from build123d import *

# Parameters (mm, degrees)
SKETCH_4_W          = 160
SKETCH_4_H          = 115
EXTRUDE_1_DEPTH     = 20
CUT_EXTRUDE_1_DEPTH = 20
SKETCH_16_R         = 5.5
CUT_EXTRUDE_2_DEPTH = 15


with BuildPart() as part:
    # 草圖4 → 填料-伸長1 (new body)
    with BuildSketch(Plane.XY):
        with Locations((14.659712787, 72.59909222)):
            Rectangle(SKETCH_4_W, SKETCH_4_H)
    extrude(amount=EXTRUDE_1_DEPTH)

    # 草圖2 → 除料-伸長1 (cut)
    with BuildSketch(Plane.XY):
        with BuildLine():
            Line((9.582154386, 114.239387395), (32.639572719, 114.239387395))
            Line((32.639572719, 114.239387395), (35.911975242, 114.239387395))
            Line((35.911975242, 114.239387395), (35.911975242, 122.748829131))
            Line((35.911975242, 122.748829131), (43.825042281, 122.748829131))
            Line((43.825042281, 122.748829131), (43.825042281, 116.150572029))
            Line((43.825042281, 116.150572029), (45.365452665, 116.150572029))
            Line((45.365452665, 116.150572029), (45.365452665, 126.787374199))
            Line((45.365452665, 126.787374199), (50.650153823, 126.787374199))
            Line((50.650153823, 126.787374199), (50.650153823, 116.150572029))
            Line((50.650153823, 116.150572029), (51.63260176, 116.150572029))
            Line((51.63260176, 116.150572029), (51.63260176, 122.748829131))
            Line((51.63260176, 122.748829131), (58.302252446, 122.748829131))
            Line((58.302252446, 122.748829131), (58.302252446, 114.239387395))
            ThreePointArc((58.302252446, 114.239387395), (68.354977159, 111.933757574), (76.3981894, 105.477757274))
            ThreePointArc((76.3981894, 105.477757274), (77.386875553, 104.202213525), (78.350890948, 102.907923572))
            ThreePointArc((78.350890948, 102.907923572), (85.469179447, 90.183153699), (89.343429579, 76.126838912))
            Line((89.343429579, 76.126838912), (89.450916797, 75.407862922))
            ThreePointArc((89.450916797, 75.407862922), (89.659712787, 72.59909222), (89.450916797, 69.790321519))
            Line((89.450916797, 69.790321519), (89.343429579, 69.071345528))
            ThreePointArc((89.343429579, 69.071345528), (85.469179447, 55.015030741), (78.350890948, 42.290260868))
            ThreePointArc((78.350890948, 42.290260868), (77.386875553, 40.995970915), (76.3981894, 39.720427166))
            ThreePointArc((76.3981894, 39.720427166), (68.354977159, 33.264426866), (58.302252446, 30.958797045))
            Line((58.302252446, 30.958797045), (58.302252446, 22.449355309))
            Line((58.302252446, 22.449355309), (51.63260176, 22.449355309))
            Line((51.63260176, 22.449355309), (51.63260176, 29.047612411))
            Line((51.63260176, 29.047612411), (50.650153823, 29.047612411))
            Line((50.650153823, 29.047612411), (50.650153823, 18.410810241))
            Line((50.650153823, 18.410810241), (45.365452665, 18.410810241))
            Line((45.365452665, 18.410810241), (45.365452665, 29.047612411))
            Line((45.365452665, 29.047612411), (43.825042281, 29.047612411))
            Line((43.825042281, 29.047612411), (43.825042281, 22.449355309))
            Line((43.825042281, 22.449355309), (35.911975242, 22.449355309))
            Line((35.911975242, 22.449355309), (35.911975242, 30.958797045))
            Line((35.911975242, 30.958797045), (32.639572719, 30.958797045))
            Line((32.639572719, 30.958797045), (9.582154386, 30.958797045))
            ThreePointArc((9.582154386, 30.958797045), (2.328045496, 31.402381927), (-4.817967678, 32.726526576))
            ThreePointArc((-4.817967678, 32.726526576), (-19.619782039, 37.212171907), (-33.900352311, 43.151871824))
            ThreePointArc((-33.900352311, 43.151871824), (-39.787433986, 46.173940455), (-45.481740166, 49.545217155))
            ThreePointArc((-45.481740166, 49.545217155), (-51.391366265, 54.573313812), (-55.677619443, 61.041193705))
            ThreePointArc((-55.677619443, 61.041193705), (-58.292337425, 72.59909222), (-55.677619443, 84.156990735))
            ThreePointArc((-55.677619443, 84.156990735), (-51.391366265, 90.624870628), (-45.481740166, 95.652967285))
            ThreePointArc((-45.481740166, 95.652967285), (-39.787433986, 99.024243985), (-33.900352311, 102.046312617))
            ThreePointArc((-33.900352311, 102.046312617), (-19.619782039, 107.986012534), (-4.817967678, 112.471657865))
            ThreePointArc((-4.817967678, 112.471657865), (2.328045496, 113.795802514), (9.582154386, 114.239387395))
        make_face()
    extrude(amount=CUT_EXTRUDE_1_DEPTH, mode=Mode.SUBTRACT)

    # 草圖16 → 除料-伸長2 (cut)
    with BuildSketch(Plane(origin=(-66.2, 0, 0), x_dir=(0, 0, -1), z_dir=(1, 0, 0))):
        with Locations((-10, 120.09909222)):
            Circle(SKETCH_16_R)
        with Locations((-10, 105.09909222)):
            Circle(SKETCH_16_R)
        with Locations((-10, 40.09909222)):
            Circle(SKETCH_16_R)
        with Locations((-10, 25.09909222)):
            Circle(SKETCH_16_R)
    extrude(amount=CUT_EXTRUDE_2_DEPTH, mode=Mode.SUBTRACT)


solid = part.part
Model file for the job. Use its own axes, mm. A direction names the side the tool comes from. Give positions to 0.01 mm unless a question says otherwise; leave off trailing zeros. Order: outer loops, then holes, each group sorted by start corner. A loop starts at its lowest first (then second) coordinate and runs counter-clockwise, first axis right, second up. Notation, with made-up numbers: (57.5, 38) -> (86.5, 38) arc R10 ccw to (86.5, 44) -> close; hole circle Ø9 at (-23, 70). An arc over 180 degrees is marked (long way). Use CSV: the item, a comma, the result in double quotes.
1. Mould opens along Y. For faces 1 (the flat face through (14, 15.099, 10)), 2 (the flat face through (43.825, 26, 10)), 3 (the flat face through (-65.34, 72, 10)) say: +Y half, -Y half, draft (parallel to the pull), parting line (faces both ways), or undercut.
Outcome:
face 1,"-Y half"
face 2,"undercut"
face 3,"draft"
2. 3-axis set-ups, long thin cutter, end or side, ignore diameter. For faces 4 (the flat face through (43.825, 119, 10)), 5 (the cylindrical face through (-58.37, 110.55, 10.72)): which of +Z, -Z, +X, -X, +Y, -Y reach the whole face in a straight line?
Outcome:
face 4,"+Z, -Z"
face 5,"-X"
3. Band-saw the part on B-B, the plane y = 55. Give the cut face in (x, z).
Outcome:
outline,"(-65.34, 0) -> (-51.76, 0) -> (-51.76, 20) -> (-65.34, 20) -> close; (85.46, 0) -> (94.66, 0) -> (94.66, 20) -> (85.46, 20) -> close"
4. Band-saw the part on A-A, the plane x = 38.5. Give the cut face in (y, z), then the cut area to 3 significant figures.
Outcome:
outline,"(15.1, 0) -> (22.45, 0) -> (22.45, 20) -> (15.1, 20) -> close; (122.75, 0) -> (130.1, 0) -> (130.1, 20) -> (122.75, 20) -> close"
area,"294 mm²"
5. Drop flat-ended pins along their axis: pin 1 (2 mm diameter, centred on y = 26, z = 14, fed in from -X); pin 2 (12 mm diameter, centred on y = 105.5, z = 12, fed in from -X). Give the stop position or say it passes through.
Outcome:
pin 1,"x = -51.2"
pin 2,"x = -65.34"
6. Drill centre lines: line 1 along Y through (x, z) = (-59.5, 10); line 2 along X through (y, z) = (120.5, 16.5); line 3 along Y through (x, z) = (-54.5, 10). Where is each one in solid material? Low to high. Write a range as from..to.
Outcome:
line 1,"15.1..19.6, 30.6..34.6, 45.6..99.6, 110.6..114.6, 125.6..130.1"
line 2,"-65.34..35.91, 43.83..45.37, 50.65..51.63, 58.3..94.66"
line 3,"15.1..19.6, 30.6..34.6, 45.6..58.83, 86.36..99.6, 110.6..114.6, 125.6..130.1"
